from build123d import *

# Parameters (mm, degrees)
SKETCH_1_W          = 190
SKETCH_1_H          = 116
SKETCH_1_W_2        = 166
SKETCH_1_H_2        = 100
EXTRUDE_2_DEPTH     = 8
SKETCH_2_W          = 190
SKETCH_2_H          = 116
SKETCH_2_W_2        = 182
SKETCH_2_H_2        = 108
EXTRUDE_3_DEPTH     = 7.5
FILLET_1_R          = 8
SKETCH_3_W          = 15
SKETCH_3_H          = 7.5
CUT_EXTRUDE_1_DEPTH = 7.5
SKETCH_4_W          = 16
SKETCH_4_H          = 3
CUT_EXTRUDE_2_DEPTH = 35.5
SKETCH_5_R          = 1.6
CUT_EXTRUDE_3_DEPTH = 35.5
CHAMFER_1_SIZE      = 1.5
CHAMFER_1_SIZE2     = 0.866025404
SKETCH_6_W          = 22
SKETCH_6_H          = 2.5
CUT_EXTRUDE_4_DEPTH = 4
FILLET_2_R          = 4


with BuildPart() as part:
    # 草图1 → 凸台-拉伸2 (new body)
    with BuildSketch(Plane(origin=(0, 0, 0), x_dir=(1, 0, 0), z_dir=(0, 1, 0))):
        Rectangle(SKETCH_1_W, SKETCH_1_H)
        Rectangle(SKETCH_1_W_2, SKETCH_1_H_2, mode=Mode.SUBTRACT)
    extrude(amount=EXTRUDE_2_DEPTH)

    # 草图2 → 凸台-拉伸3 (add)
    with BuildSketch(Plane.XZ):
        Rectangle(SKETCH_2_W, SKETCH_2_H)
        Rectangle(SKETCH_2_W_2, SKETCH_2_H_2, mode=Mode.SUBTRACT)
    extrude(amount=EXTRUDE_3_DEPTH)

    # 圆角1
    fillet_1_edges = [part.edges().sort_by_distance(p)[0] for p in [
        (-95, 0.25, 58),
        (95, 0.25, 58),
        (95, 0.25, -58),
        (-95, 0.25, -58),
    ]]
    fillet(fillet_1_edges, radius=FILLET_1_R)

    # 草图3 → 切除-拉伸1 (cut)
    with BuildSketch(Plane.ZY.offset(95)):
        with Locations((0, -3.75)):
            Rectangle(SKETCH_3_W, SKETCH_3_H)
    extrude(amount=-CUT_EXTRUDE_1_DEPTH, mode=Mode.SUBTRACT)

    # 草图4 → 切除-拉伸2 (cut)
    with BuildSketch(Plane(origin=(0, 0, -58), x_dir=(-1, 0, 0), z_dir=(0, 0, -1))):
        with Locations((-62, -2.5)):
            Rectangle(SKETCH_4_W, SKETCH_4_H)
    extrude(amount=-CUT_EXTRUDE_2_DEPTH, mode=Mode.SUBTRACT)

    # 草图5 → 切除-拉伸3 (cut)
    with BuildSketch(Plane(origin=(0, 8, 0), x_dir=(1, 0, 0), z_dir=(0, 1, 0))):
        with Locations(Location((-87.4, 50.9, 0), (0, 0, 270))):
            Circle(SKETCH_5_R)
        with Locations(Location((-87.4, -50.9, 0), (0, 0, 90))):
            Circle(SKETCH_5_R)
        with Locations(Location((87.4, -50.9, 0), (0, 0, 270))):
            Circle(SKETCH_5_R)
        with Locations(Location((87.4, 50.9, 0), (0, 0, 90))):
            Circle(SKETCH_5_R)
    extrude(amount=-CUT_EXTRUDE_3_DEPTH, mode=Mode.SUBTRACT)

    # 倒角1
    chamfer_1_edges = [part.edges().sort_by_distance(p)[0] for p in [
        (87.4, 8, -49.3),
        (87.4, 8, 49.3),
        (-87.4, 8, 52.5),
        (-87.4, 8, -52.5),
    ]]
    chamfer_1_side = [part.faces().sort_by_distance(p)[0] for p in [
        (0, 8, -55.773882303),
    ]]
    chamfer(chamfer_1_edges, length=CHAMFER_1_SIZE, length2=CHAMFER_1_SIZE2, reference=chamfer_1_side[0])

    # 草图6 → 切除-拉伸4 (cut)
    with BuildSketch(Plane.ZY.offset(95)):
        with Locations((-32.5, -6.35)):
            Rectangle(SKETCH_6_W, SKETCH_6_H)
    extrude(amount=-CUT_EXTRUDE_4_DEPTH, mode=Mode.SUBTRACT)

    # 圆角2
    fillet_2_edges = [part.edges().sort_by_distance(p)[0] for p in [
        (95, 8, 0),
        (0, 8, 58),
        (-95, 8, 0),
        (0, 8, -58),
        (-92.656854249, 8, 55.656854249),
        (-92.656854249, 8, -55.656854249),
        (92.656854249, 8, -55.656854249),
        (92.656854249, 8, 55.656854249),
    ]]
    fillet(fillet_2_edges, radius=FILLET_2_R)


solid = part.part
CAD build for the part. Positions are in the model's coordinates, mm. A direction names the side the tool comes from. Coordinates: 2 decimals unless noted, no trailing zeros. Write each loop counter-clockwise with the first axis right and the second up, starting at its lowest first coordinate (ties: lowest second). Pieces come first, ordered by that corner, then holes. Notation, with made-up numbers: (6, 75) - (51, 75) arc R23 ccw to (51, 112) - close; hole circle Ø4 at (17.25, -2). An arc over 180 degrees is marked (long way). Use a Markdown table: item, result. Add a question column.
Item 1: Mould opens along Z. For faces 5 (the face through (92.594, -1.83, -55.719)), 6 (the face through (62, -4, -56)), 7 (the face through (-1, -4, -54)) say: pulls with the +Z half, pulls with the -Z half, needs draft (parallel to the pull), parting line crosses it, or undercut.
Item 2: Drill centre lines: L1, parallel to X at y = 3, z = -39; L2, parallel to Z at x = 64, y = 1.5; L3, parallel to X at y = -5.5, z = 10.5. Where is each one in solid material? Low to high. Write a range as from..to.
Item 3: Flat gauge pins, fed straight in: pin 1 (9 mm diameter, centred on y = 4.5, z = 23.5, fed in from +X); pin 2 (6 mm diameter, centred on y = -4, z = 1, fed in from -X); pin 3 (1.5 mm diameter, centred on y = -2.5, z = -55.5, fed in from +X); pin 4 (1.2 mm diameter, centred on x = 61, z = -55, fed in from +Y). Where does each tip first touch, or does it go through?
Item 4: 3-axis set-ups, long thin cutter, end or side, ignore diameter. For faces 1 (the face through (-83, 4, 1)), 2 (the face through (-93, -4, 7.5)), 3 (the face through (-93, -7.5, -14)), 4 (the face through (-1, -4, 54)): which of +Z, -Z, +X, -X, +Y, -Y reach the whole face in a straight line?
Item 5: Band-saw the part on A-A, the plane z = 2. Give the cut face in (x, y).
Numbers:
| question | item | result |
|---|---|---|
| 1 | face 5 | pulls with the -Z half |
| 1 | face 6 | needs draft |
| 1 | face 7 | undercut |
| 2 | L1 | -95..-83, 83..95 |
| 2 | L2 | -58..-50, 50..58 |
| 2 | L3 | -95..-91, 91..95 |
| 3 | pin 1 | x = 95 |
| 3 | pin 2 | x = 91 |
| 3 | pin 3 | x = 93.44 |
| 3 | pin 4 | y = 7.98 |
| 4 | face 1 | +Y, -Y |
| 4 | face 2 | -X, -Y |
| 4 | face 3 | +Z, -Z, +X, -X, -Y |
| 4 | face 4 | -Y |
| 5 | outline | (-95, 0) - (-83, 0) - (-83, 8) - (-91, 8) arc R4 ccw to (-95, 4) - close; (83, 0) - (91, 0) - (91, -7.5) - (95, -7.5) - (95, 4) arc R4 ccw to (91, 8) - (83, 8) - close |
